Part model, mm, in its own coordinate system. A direction names the side the tool comes from. Coordinates: 2 decimals unless noted, no trailing zeros. Loops run counter-clockwise (first coordinate to the right, second up) from the corner with the lowest first, then second, coordinate; pieces in that order, holes last. Notation, with made-up numbers: (56, 56) -> (63, 56) arc R28 ccw to (63, 89) -> close; hole circle Ø7 at (70, -1). An arc over 180 degrees is marked (long way). One line per item, written item: value. Start each with the question number.
from build123d import *

# Parameters (mm, degrees)
SKETCH2_OUTSIDE_W   = 31.923
SKETCH2_OUTSIDE_H   = 31.922
SKETCH2_OUTSIDE_W_2 = 16.752450568
SKETCH2_OUTSIDE_H_2 = 14.605
CUT_EXTRUDE1_DEPTH  = 10.287
SKETCH3_OUTSIDE_W   = 22.89
SKETCH3_OUTSIDE_H   = 30.51
SKETCH3_OUTSIDE_W_2 = 14.605
SKETCH3_OUTSIDE_H_2 = 16.752450568
CUT_EXTRUDE3_DEPTH  = 11.303
SKETCH6_R           = 6.35
CUT_EXTRUDE4_DEPTH  = 2.54
CUT_EXTRUDE4_TAPER  = 30
BOSS_EXTRUDE1_DEPTH = 8.636
BOSS_EXTRUDE2_DEPTH = 8.636
BOSS_EXTRUDE3_DEPTH = 8.636
BOSS_EXTRUDE4_DEPTH = 8.636


with BuildPart() as part:
    # Sketch1 → Revolve1 (revolve)
    with BuildSketch(Plane(origin=(0, 0, 0), x_dir=(1, 0, 0), z_dir=(0, 1, 0))):
        with BuildLine():
            Line((0, 11.1125), (0, -11.1125))
            ThreePointArc((0, -11.1125), (11.1125, 0), (0, 11.1125))
        make_face()
    revolve(axis=Axis((0, 0, 7.836824486), (0, 0, -1)))

    # Sketch2 outside → Cut-Extrude1 (cut, symmetric)
    with BuildSketch(Plane(origin=(0, 0, 0), x_dir=(1, 0, 0), z_dir=(0, 1, 0))):
        with Locations((-0.0005, 0)):
            Rectangle(SKETCH2_OUTSIDE_W, SKETCH2_OUTSIDE_H)
        Rectangle(SKETCH2_OUTSIDE_W_2, SKETCH2_OUTSIDE_H_2, mode=Mode.SUBTRACT)
    extrude(amount=CUT_EXTRUDE1_DEPTH, both=True, mode=Mode.SUBTRACT)

    # Sketch3 outside → Cut-Extrude3 (cut, symmetric)
    with BuildSketch(Plane(origin=(0, 0, 0), x_dir=(0, 0, -1), z_dir=(1, 0, 0))):
        Rectangle(SKETCH3_OUTSIDE_W, SKETCH3_OUTSIDE_H)
        Rectangle(SKETCH3_OUTSIDE_W_2, SKETCH3_OUTSIDE_H_2, mode=Mode.SUBTRACT)
    extrude(amount=CUT_EXTRUDE3_DEPTH, both=True, mode=Mode.SUBTRACT)

    # Sketch6 → Cut-Extrude4 (cut)
    with BuildSketch(Plane.XY.offset(7.3025)):
        Circle(SKETCH6_R)
    cut_extrude4 = extrude(amount=-CUT_EXTRUDE4_DEPTH, taper=CUT_EXTRUDE4_TAPER, mode=Mode.SUBTRACT)

    # Mirror1: Cut-Extrude4 across plane
    add(cut_extrude4.mirror(Plane.XY), mode=Mode.SUBTRACT)

    # Sketch7 → Boss-Extrude1 (add)
    with BuildSketch(Plane(origin=(8.376225284, 0, 0), x_dir=(0, 0, -1), z_dir=(1, 0, 0))):
        with BuildLine():
            ThreePointArc((7.3025, 0), (0, 7.3025), (-7.3025, 0))
            ThreePointArc((-7.3025, 0), (0, -7.3025), (7.3025, 0))
        make_face()
    extrude(amount=BOSS_EXTRUDE1_DEPTH)

    # Sketch11 → Boss-Extrude2 (add)
    with BuildSketch(Plane(origin=(0, 8.376225284, 0), x_dir=(1, 0, 0), z_dir=(0, 1, 0))):
        with BuildLine():
            ThreePointArc((0, -7.3025), (7.3025, 0), (0, 7.3025))
            ThreePointArc((0, 7.3025), (-7.3025, 0), (0, -7.3025))
        make_face()
    extrude(amount=BOSS_EXTRUDE2_DEPTH)

    # Sketch12 → Boss-Extrude3 (add)
    with BuildSketch(Plane.ZY.offset(8.376225284)):
        with BuildLine():
            ThreePointArc((7.3025, 0), (0, 7.3025), (-7.3025, 0))
            ThreePointArc((-7.3025, 0), (0, -7.3025), (7.3025, 0))
        make_face()
    extrude(amount=BOSS_EXTRUDE3_DEPTH)

    # Sketch13 → Boss-Extrude4 (add)
    with BuildSketch(Plane.XZ.offset(8.376225284)):
        with BuildLine():
            ThreePointArc((0, -7.3025), (7.3025, 0), (0, 7.3025))
            ThreePointArc((0, 7.3025), (-7.3025, 0), (0, -7.3025))
        make_face()
    extrude(amount=BOSS_EXTRUDE4_DEPTH)


solid = part.part
1) Slice it at C-C (z = 0). Give the cut face in (x, y) (1 decimal).
2) Pin check, flat tips, straight feed: pin 1 Ø5 at (x, y) = (0, -0.5) entering from -Z; pin 2 Ø5 at (x, y) = (-10.5, 5) entering from +Z; pin 3 Ø6 at (x, z) = (-11.5, -0.5) entering from +Y. Stop position of each tip, or through.
3) Slice it at A-A (z = 6.25). Give the cut face in (x, y).
4) Tool access for faces 4 (the flat face through (0, 0, -4.762)), 5 (the flat face through (0, 0, 4.762)), 6 (the cylindrical face through (-12.63, -7.24, 0.95)), 7 (the cylindrical face through (-7.24, 12.63, 0.95)), 8 (the cylindrical face through (12.63, -7.24, -0.95)): list every direction of +Z, -Z, +X, -X, +Y, -Y with a clear straight run to the whole face (end or side of a thin tool).
5) Probe line 1 (Z direction, x = -1, y = -2); line 2 (X direction, y = 9, z = 0); line 3 (Y direction, x = 1.5, z = 6.75). List the from-to ranges inside material, lowest first. Write a range as from..to.
6) Slice it at B-B (x = 11.5). Give the cut face in (y, z) (1 decimal), then the cut area to 3 significant figures.
7) Pull direction X, two halves, no side cores. Call faces 1 (the conical face through (2.3, -4.4, -4.9)), 2 (the cylindrical face through (-7.24, -12.63, -0.95)), 3 (the flat face through (0, -17.012, 0)): +X half, -X half, draft (parallel to the pull), parting line (faces both ways), or undercut.
Check sheet entries:
1. outline: (-17, -7.3) -> (-8.4, -7.3) arc R11.1 ccw to (-7.3, -8.4) -> (-7.3, -17) -> (7.3, -17) -> (7.3, -8.4) arc R11.1 ccw to (8.4, -7.3) -> (17, -7.3) -> (17, 7.3) -> (8.4, 7.3) arc R11.1 ccw to (7.3, 8.4) -> (7.3, 17) -> (-7.3, 17) -> (-7.3, 8.4) arc R11.1 ccw to (-8.4, 7.3) -> (-17, 7.3) -> close
2. pin 1: stops at z = -4.76
2. pin 2: stops at z = 6.86
2. pin 3: stops at y = 7.3
3. outline: (-17.01, -3.78) -> (-8.38, -3.78) arc R9.19 ccw to (-3.78, -8.38) -> (-3.78, -17.01) -> (3.78, -17.01) -> (3.78, -8.38) arc R9.19 ccw to (8.38, -3.78) -> (17.01, -3.78) -> (17.01, 3.78) -> (8.38, 3.78) arc R9.19 ccw to (3.78, 8.38) -> (3.78, 17.01) -> (-3.78, 17.01) -> (-3.78, 8.38) arc R9.19 ccw to (-8.38, 3.78) -> (-17.01, 3.78) -> close; hole circle Ø11.48 at (0, 0)
4. face 4: -Z
4. face 5: +Z
4. face 6: -X
4. face 7: +Y
4. face 8: +X
5. line 1: z = -4.76..4.76
5. line 2: x = -7.3..7.3
5. line 3: y = -17.01..-5.84, 5.84..17.01
6. outline: circle Ø14.6 at (0, 0)
6. area: 168 mm^2
7. face 1: undercut
7. face 2: parting line
7. face 3: draft
